Check sheet for the modelled part. Datum: model origin and axes. Units: mm. A direction names the side the tool comes from. Coordinates: 2 decimals unless noted, no trailing zeros. Write each loop counter-clockwise with the first axis right and the second up, starting at its lowest first coordinate (ties: lowest second). Pieces come first, ordered by that corner, then holes. Notation, with made-up numbers: M -34.75,40.25 L 23.25,40.25 A23 cw 23.25,67.25 Z; hole C -39,47.25 d8. An arc over 180 degrees is marked long. Answer as CSV lines item,"result". Start each with the question number.
Q1. Thickness scan on line 1 along Z through (x, y) = (0.5, -3.5); line 2 along X through (y, z) = (0, 27) (3 decimals); line 3 along Y through (x, z) = (-3, 30). Record the ranges inside material, lowest first. Write a range as from..to.
Q2. Sectioned sample at D-D, the plane z = 42. Record the cut outline in (x, y), then the cut area to 3 significant figures.
Q3. Depth check by flat-ended pin: pin 1 Ø4 at (y, z) = (4, 38.5) entering from -X; pin 2 Ø1.5 at (x, z) = (-5.5, 23.5) entering from +Y; pin 3 Ø1 at (y, z) = (2, 42.5) entering from -X. Enter the tip coordinate at first touch or a pass-through.
Q4. Sectioned sample at B-B, the plane y = 0. Record the cut outline in (x, z).
Q5. Access from +Z, -Z, +X, -X, +Y, -Y to the whole of each face (thin tool, end or side, straight path). Record for faces 4 (the flat face through (0, 0, 40)), 5 (the flat face through (4, -8, 40)), 6 (the flat face through (-3, -3, 0)).
Q6. Sectioned sample at A-A, the plane z = 14. Record the cut outline in (x, y).
Q7. Mould release check, pull along Z, two halves, no side actions. Record for faces 1 (the conical face through (8.554, 2.694, 21.266)), 2 (the flat face through (0, 0, 50)), 3 (the cylindrical face through (-1.5, 11.4, 44.1)): pulls with the +Z half, pulls with the -Z half, needs draft (parallel to the pull), parting line crosses it, or undercut.
from build123d import *

# Parameters (mm, degrees)
F2_SIZE  = 2
F3_SIZE  = 2
F4_R     = 4
F5_DEPTH = 40


with BuildPart() as f1:
    # F0 (on Front) → F1 (revolve)
    with BuildSketch(Plane.XZ):
        Polygon((0, 40), (0, 0), (9.5, 0), (8.5, 40), (11.5, 40), (11.5, 50), (8.5, 50), (0, 50), align=None)
    revolve(axis=Axis((0, 0, 45), (0, 0, 1)))

    # F2
    f2_edges = [f1.edges().sort_by_distance(p)[0] for p in [
        (-9.5, 0, 0),
    ]]
    chamfer(f2_edges, length=F2_SIZE)

    # F3
    f3_edges = [f1.edges().sort_by_distance(p)[0] for p in [
        (-11.5, 0, 50),
    ]]
    chamfer(f3_edges, length=F3_SIZE)

    # F4 (on face) → F5 (cut, through all)
    with BuildSketch(Plane(origin=(0, 0, 0), x_dir=(1, 0, 0), z_dir=(0, 0, -1))):
        Circle(F4_R)
    extrude(amount=-F5_DEPTH, mode=Mode.SUBTRACT)


solid = f1.part
Output:
1,line 1,"z = 40..50"
1,line 2,"x = -8.825..-4, 4..8.825"
1,line 3,"y = -8.22..-2.65, 2.65..8.22"
2,outline,"C 0,0 d23"
2,area,"415 mm^2"
3,pin 1,"stops at x = -11.18"
3,pin 2,"stops at y = 7.54"
3,pin 3,"stops at x = -11.4"
4,outline,"M -11.5,40 L -8.5,40 L -9.45,2 L -7.5,0 L -4,0 L -4,40 L 4,40 L 4,0 L 7.5,0 L 9.45,2 L 8.5,40 L 11.5,40 L 11.5,48 L 9.5,50 L -9.5,50 L -11.5,48 Z"
5,face 4,"-Z"
5,face 5,"none"
5,face 6,"-Z, +X, -X, +Y, -Y"
6,outline,"C 0,0 d18.3; hole C 0,0 d8"
7,face 1,"undercut"
7,face 2,"pulls with the +Z half"
7,face 3,"needs draft"
